Solid Edge part; units mm, degrees
sketch "Sketch1" plane through (0, 0, 0) normal (0, -1, 0) x (1, 0, 0)
  circle A0 centre (0, 0) radius 11
  circle A1 centre (0, 0) radius 4
extrude "Protrusion1" add sketch "Sketch1" against normal blind 7
sketch "Sketch2" plane through (0, 0, 0) normal (0, -1, 0) x (1, 0, 0)
  circle A0 centre (0, 0) radius 8.6
  circle A1 centre (0, 0) radius 6.3
extrude "ExtrudedCutout_1" cut sketch "Sketch2" against normal blind 1
sketch "Sketch3" plane through (0, 7, 0) normal (0, 1, 0) x (-1, 0, 0)
  circle A0 centre (0, 0) radius 8.6
  circle A1 centre (0, 0) radius 6.3
extrude "ExtrudedCutout_3" cut sketch "Sketch3" against normal blind 0.5
properties material "Steel"
Geometry check sheet. Reference: the model listing, model coordinates, mm. A direction names the side the tool comes from. Round coordinates to 2 decimals unless told otherwise and drop trailing zeros. Order: outer loops, then holes, each group sorted by start corner. A loop starts at its lowest first (then second) coordinate and runs counter-clockwise, first axis right, second up. Notation, with made-up numbers: (-22, 0.25) - (-10, 0.25) arc R22 ccw to (-10, 6.25) - close; hole circle Ø5 at (52.25, 13.25). An arc over 180 degrees is marked (long way). Use a Markdown table: item, result. Add a question column.
1) Gauge pin test, flat ends, axial feed: P1, Ø2, axis at x = -1, y = 5, coming from the -Z side; P2, Ø1.5, axis at y = 3.5, z = -4, coming from the -X side. Record the tip position at first contact, or that the pin passes through.
2) Section check A-A (z = 0). Record the cut outline in (x, y), then the cut area to 3 significant figures.
3) Section check D-D (y = 3.25). Record the cut outline in (x, z).
4) Thickness scan on line 1 along Z through (x, y) = (0, 6.7); line 2 along Z through (x, y) = (0, 4); line 3 along Y through (x, z) = (-8, -0.5). Record the ranges inside material, lowest first.
5) Set-up check for faces 1 (the cylindrical face through (5, 6.75, -3.83)), 2 (the flat face through (-6, 7, 7)), 3 (the flat face through (3, 1, 6)): record each of +Z, -Z, +X, -X, +Y, -Y from which the full face is reachable in a straight line by a thin tool's end or side.
6) Section check B-B (x = 0). Record the cut outline in (y, z), then the cut area to 3 significant figures.
7) Section check C-C (y = 0.5). Record the cut outline in (x, z), then the cut area to 3 significant figures.
8) Mould release check, pull along X, two halves, no side actions. Record for faces 4 (the flat face through (-6, 0, 7)), 5 (the cylindrical face through (-2.38, 3.45, -10.74)), 6 (the cylindrical face through (8.59, 6.75, 0.38)): released by +X, released by -X, zero draft, split by the parting line, or undercut.
Established:
| question | item | result |
|---|---|---|
| 1 | P1 | z = -11 |
| 1 | P2 | x = -10.51 |
| 2 | outline | (-11, 0) - (-8.6, 0) - (-8.6, 1) - (-6.3, 1) - (-6.3, 0) - (-4, 0) - (-4, 7) - (-6.3, 7) - (-6.3, 6.5) - (-8.6, 6.5) - (-8.6, 7) - (-11, 7) - close; (4, 0) - (6.3, 0) - (6.3, 1) - (8.6, 1) - (8.6, 0) - (11, 0) - (11, 7) - (8.6, 7) - (8.6, 6.5) - (6.3, 6.5) - (6.3, 7) - (4, 7) - close |
| 2 | area | 91.1 mm2 |
| 3 | outline | circle Ø22 at (0, 0); hole circle Ø8 at (0, 0) |
| 4 | line 1 | -11 to -8.6, -6.3 to -4, 4 to 6.3, 8.6 to 11 |
| 4 | line 2 | -11 to -4, 4 to 11 |
| 4 | line 3 | 1 to 6.5 |
| 5 | face 1 | +Y |
| 5 | face 2 | +Z, -Z, +X, -X, +Y |
| 5 | face 3 | -Y |
| 6 | outline | (0, -11) - (7, -11) - (7, -8.6) - (6.5, -8.6) - (6.5, -6.3) - (7, -6.3) - (7, -4) - (0, -4) - (0, -6.3) - (1, -6.3) - (1, -8.6) - (0, -8.6) - close; (0, 4) - (7, 4) - (7, 6.3) - (6.5, 6.3) - (6.5, 8.6) - (7, 8.6) - (7, 11) - (0, 11) - (0, 8.6) - (1, 8.6) - (1, 6.3) - (0, 6.3) - close |
| 6 | area | 91.1 mm2 |
| 7 | outline | circle Ø22 at (0, 0); circle Ø12.6 at (0, 0); hole circle Ø17.2 at (0, 0); hole circle Ø8 at (0, 0) |
| 7 | area | 222 mm2 |
| 8 | face 4 | zero draft |
| 8 | face 5 | split by the parting line |
| 8 | face 6 | undercut |
